from build123d import *


# Not quite as in the source:
# - a feature names something its author has since deleted; it is built from what else it names


with BuildPart() as f1:
    # F0 (on Front) → F1 (revolve)
    with BuildSketch(Plane.XZ):
        with BuildLine():
            Line((0, 7.540625), (0, 12.2555))
            Line((0, 12.2555), (-8.7592504682, 9.9084659107))
            ThreePointArc((-8.7592504682, 9.9084659107), (-10.4563968554, 8.7744689494), (-11.1125, 6.8416514123))
            Line((-11.1125, 6.8416514123), (-11.1125, 6.49986))
            Line((-11.1125, 6.49986), (-6.35, 6.49986))
            Line((-6.35, 6.49986), (-6.35, 7.540625))
            Line((-6.35, 7.540625), (0, 7.540625))
        make_face()
    revolve(axis=Axis((5.2561350167, 0, 0), (1, 0, 0)))


solid = f1.part
Model file for the job. Use its own axes, mm. Round coordinates to 2 decimals unless told otherwise and drop trailing zeros. Order: outer loops, then holes, each group sorted by start corner. A loop starts at its lowest first (then second) coordinate and runs counter-clockwise, first axis right, second up.
(1) Pull direction Z, two halves, no side cores. Call faces 1 (the face through (0, 5, 6)), 2 (the face through (-6.35, -6, -3)), 3 (the face through (-8.698, -5.481, 3.494)), 4 (the face through (-7.36, 10.04, -2.23)): released by +Z, released by -Z, zero draft, split by the parting line, or undercut.
(2) Drill centre lines: line 1 (Y direction, x = -5.5, z = 3); line 2 (Z direction, x = -10.1, y = 0); line 3 (Y direction, x = -1.25, z = 0). Where is each one in solid material? Low to high.
(3) Band-saw the part on C-C (x = -5). List the corners of the cut face in (y, z).
(4) Band-saw the part on D-D (x = -2.75). List the corners of the cut face in (y, z), then the cut area to 3 significant figures.
(5) Pin check, flat tips, straight feed: pin 1 (4 mm diameter, centred on x = -8.5, z = 3.5, fed in from -Y); pin 2 (11.5 mm diameter, centred on y = 0, z = 0, fed in from +X); pin 3 (4 mm diameter, centred on x = -8.5, z = 0.5, fed in from -Y); pin 4 (5 mm diameter, centred on x = -9, y = 7.5, fed in from +Z). Stop position of each tip, or through.
Verdict:
1. face 1: zero draft
1. face 2: undercut
1. face 3: undercut
1. face 4: split by the parting line
2. line 1: y = -10.36 to -6.92, 6.92 to 10.36
2. line 2: z = -9.17 to -6.5, 6.5 to 9.17
2. line 3: y = -11.92 to -7.54, 7.54 to 11.92
3. outline: circle Ø21.83 at (0, 0); hole circle Ø15.08 at (0, 0)
4. outline: circle Ø23.04 at (0, 0); hole circle Ø15.08 at (0, 0)
4. area: 238 mm2
5. pin 1: stops at y = -10.15
5. pin 2: passes through
5. pin 3: stops at y = -10.51
5. pin 4: stops at z = 8.67
